from build123d import *

# Parameters (mm, degrees)
SKETCH1_R           = 18
BOSS_EXTRUDE1_DEPTH = 50
SKETCH2_R           = 1.5
BOSS_EXTRUDE2_DEPTH = 17
SKETCH3_W           = 19
SKETCH3_H           = 8.5
BOSS_EXTRUDE3_DEPTH = 24
SKETCH4_R           = 1.5
CUT_EXTRUDE1_DEPTH  = 5


with BuildPart() as part:
    # Sketch1 → Boss-Extrude1 (new body)
    with BuildSketch(Plane.XY):
        Circle(SKETCH1_R)
    extrude(amount=BOSS_EXTRUDE1_DEPTH)

    # Sketch2 → Boss-Extrude2 (add)
    with BuildSketch(Plane.XY.offset(50)):
        Circle(SKETCH2_R)
    extrude(amount=BOSS_EXTRUDE2_DEPTH)

    # Sketch3 → Boss-Extrude3 (add)
    with BuildSketch(Plane(origin=(0, 0, 0), x_dir=(1, 0, 0), z_dir=(0, 1, 0))):
        with Locations((0, -4.25)):
            Rectangle(SKETCH3_W, SKETCH3_H)
    extrude(amount=BOSS_EXTRUDE3_DEPTH)

    # Sketch4 → Cut-Extrude1 (cut)
    with BuildSketch(Plane.XY.offset(50)):
        with Locations((12.5, 0)):
            Circle(SKETCH4_R)
        with Locations((6.25, -10.825317547)):
            Circle(SKETCH4_R)
        with Locations((-6.25, -10.825317547)):
            Circle(SKETCH4_R)
        with Locations((-12.5, 0)):
            Circle(SKETCH4_R)
        with Locations((-6.25, 10.825317547)):
            Circle(SKETCH4_R)
        with Locations((6.25, 10.825317547)):
            Circle(SKETCH4_R)
    extrude(amount=-CUT_EXTRUDE1_DEPTH, mode=Mode.SUBTRACT)


solid = part.part
Could you check a few things on this model? Use its own coordinates, in mm. A direction names the side the tool comes from. Round coordinates to 2 decimals unless told otherwise and drop trailing zeros. Write each loop counter-clockwise with the first axis right and the second up, starting at its lowest first coordinate (ties: lowest second). Pieces come first, ordered by that corner, then holes. Notation, with made-up numbers: (36, 82.25) - (93, 82.25) arc R33 cw to (93, 121.25) - close; hole circle Ø5 at (68, 56). An arc over 180 degrees is marked (long way). Put each result on its own line as item: value. Start each with the question number.
(1) I want a section at A-A, the plane x = 0. Please give me the cut outline in (y, z).
(2) Thinking about a two-plate mould opening in X: for faces 1 (the flat face through (-13, 0, 45)), 2 (the flat face through (6, -11, 45)), 3 (the cylindrical face through (-3.902, -17.572, 24.65)), 4 (the flat face through (9.5, 20, 4)), which applies, released by +X, released by -X, zero draft, split by the parting line, or undercut?
(3) I want a section at B-B, the plane y = 0. Please give me the cut outline in (x, z), plus the area to 3 significant figures.
(4) For faces 5 (the flat face through (-9.5, 20, 4)), 6 (the flat face through (0, 24, 4)), 7 (the cylindrical face through (11, 0, 48)), which set-ups out of +Z, -Z, +X, -X, +Y, -Y let a thin tool reach every point of the face, with its end or its side?
(5) I want a section at D-D, the plane x = 6.25. Please give me the cut outline in (y, z), plus the area to 3 significant figures.
(6) I want a section at C-C, the plane z = 51.5. Please give me the cut outline in (x, y), plus the area to 3 significant figures.
(7) Will these pins go through, and if not, where does the flat tip stop? pin 1 (2.5 mm diameter, centred on x = 6.25, y = 10.83, fed in from -Z); pin 2 (3 mm diameter, centred on y = 15.5, z = 38.5, fed in from +X); pin 3 (6 mm diameter, centred on x = 4.5, z = 30, fed in from +Y); pin 4 (4 mm diameter, centred on y = 19.5, z = 52, fed in from -X).
(8) I need wall thicknesses on probe 1 along Y at (x, z) = (6, 47); probe 2 along Y at (x, z) = (-6.25, 48); probe 3 along Z at (x, y) = (2, 15.5). Which ranges of each line are inside material? Lowest first, please.
Here are the results:
1. outline: (-18, 0) - (24, 0) - (24, 8.5) - (18, 8.5) - (18, 50) - (1.5, 50) - (1.5, 67) - (-1.5, 67) - (-1.5, 50) - (-18, 50) - close
2. face 1: undercut
2. face 2: undercut
2. face 3: split by the parting line
2. face 4: released by +X
3. outline: (-18, 0) - (18, 0) - (18, 50) - (14, 50) - (14, 45) - (11, 45) - (11, 50) - (1.5, 50) - (1.5, 67) - (-1.5, 67) - (-1.5, 50) - (-11, 50) - (-11, 45) - (-14, 45) - (-14, 50) - (-18, 50) - close
3. area: 1,820 mm^2
4. face 5: +Z, -Z, -X, +Y
4. face 6: +Z, -Z, +X, -X, +Y
4. face 7: +Z
5. outline: (-16.88, 0) - (24, 0) - (24, 8.5) - (16.88, 8.5) - (16.88, 50) - (12.33, 50) - (12.33, 45) - (9.33, 45) - (9.33, 50) - (-9.33, 50) - (-9.33, 45) - (-12.33, 45) - (-12.33, 50) - (-16.88, 50) - close
5. area: 1,720 mm^2
6. outline: circle Ø3 at (0, 0)
6. area: 7.07 mm^2
7. pin 1: stops at z = 0
7. pin 2: stops at x = 11.31
7. pin 3: stops at y = 17.94
7. pin 4: passes through
8. probe 1: y = -16.97 to -12.3, -9.35 to 9.35, 12.3 to 16.97
8. probe 2: y = -16.88 to -12.33, -9.33 to 9.33, 12.33 to 16.88
8. probe 3: z = 0 to 50
